Part model, mm, in its own coordinate system. A direction names the side the tool comes from. Round coordinates to 2 decimals unless told otherwise and drop trailing zeros. Loops run counter-clockwise (first coordinate to the right, second up) from the corner with the lowest first, then second, coordinate; pieces in that order, holes last. Notation, with made-up numbers: M -37,73 L -1,73 A6 ccw -1,79 Z; hole C 54,43 d10. An arc over 180 degrees is marked long. Put each result on its own line as item: value. Start each with the question number.
1) Slice it at A-A on y = 25.5. Give the cut face in (x, z) (3 decimals).
2) Slice it at C-C on z = 19.5. Give the cut face in (x, y), then the cut area to 3 significant figures.
3) Drop flat-ended pins along their axis: pin 1 Ø2 at (y, z) = (-5, 16.5) entering from +X; pin 2 Ø5 at (x, y) = (-6.5, 16) entering from +Z (3 decimals); pin 3 Ø1.1 at (y, z) = (25, 14.5) entering from -X (3 decimals). Give the stop position or say it passes through.
4) Which spindle directions (+Z, -Z, +X, -X, +Y, -Y) get a long thin tool onto all of the face, cutting with end or side? Do faces 4 (the flat face through (10.671, 6, 5)), 5 (the flat face through (-3.81, -5, 16)), 6 (the flat face through (-8.255, 25, 13)), 7 (the cylindrical face through (9.592, 25.453, 8.452)), 8 (the cylindrical face through (-7.205, -4.454, 13.832)). Say none if no direction does.
5) Pull direction Y, two halves, no side cores. Call faces 1 (the cylindrical face through (0.14, 25.41, 12.07)), 2 (the cylindrical face through (2.736, 23.264, 21.839)), 3 (the flat face through (0, 29.21, 6)): +Y half, -Y half, draft (parallel to the pull), parting line (faces both ways), or undercut.
6) Probe line 1 along Y through (x, z) = (8.5, 4.25); line 2 along Y through (x, z) = (6.35, 2.25); line 3 along X through (y, z) = (26, 15.25) (3 decimals). List the from-to ranges inside material, lowest first.
7) Slice it at D-D on y = 21. Give the cut face in (x, z) (3 decimals).
8) Slice it at B-B on y = 5. Give the cut face in (x, z) (3 decimals).
```python
from build123d import *

# Parameters (mm, degrees)
SKETCH1_W           = 25.4
SKETCH1_H           = 35.56
SKETCH1_R           = 2.38125
BOSS_EXTRUDE1_DEPTH = 3.175
SKETCH7_W           = 25.4
SKETCH7_H           = 2.54
SKETCH7_H_2         = 7.62
BOSS_EXTRUDE3_DEPTH = 20.32
SKETCH11_R          = 1.5875
CUT_EXTRUDE1_DEPTH  = 10
CHAMFER2_SIZE       = 1.27
SKETCH13_R          = 3.175
CUT_EXTRUDE2_DEPTH  = 12.7
SKETCH14_R          = 7.14375
CUT_EXTRUDE3_DEPTH  = 3.302
CUT_EXTRUDE4_START  = -3.302
SKETCH15_R          = 7.14375
CUT_EXTRUDE4_DEPTH  = 3.302
CUT_EXTRUDE5_DEPTH  = 12.7
SKETCH17_W          = 2.029010409
SKETCH17_H          = 25.4
BOSS_EXTRUDE4_DEPTH = 12.7
CUT_EXTRUDE6_DEPTH  = 46.281333074


with BuildPart() as part:
    # Sketch1 → Boss-Extrude1 (new body)
    with BuildSketch(Plane.XY):
        with Locations((0, 11.43)):
            Rectangle(SKETCH1_W, SKETCH1_H)
        with Locations((-6.35, 3.175)):
            Circle(SKETCH1_R, mode=Mode.SUBTRACT)
        with Locations(Location((6.35, 3.175, 0), (0, 0, 180))):
            Circle(SKETCH1_R, mode=Mode.SUBTRACT)
    extrude(amount=BOSS_EXTRUDE1_DEPTH)

    # Sketch7 → Boss-Extrude3 (add)
    with BuildSketch(Plane.XY.offset(3.175)):
        with Locations((0, -5.08)):
            Rectangle(SKETCH7_W, SKETCH7_H)
        with Locations((0, 25.4)):
            Rectangle(SKETCH7_W, SKETCH7_H_2)
    extrude(amount=BOSS_EXTRUDE3_DEPTH)

    # Sketch11 → Cut-Extrude1 (cut)
    with BuildSketch(Plane.XZ.offset(6.35)):
        with Locations((-7.9375, 15.24)):
            Circle(SKETCH11_R)
        with Locations((7.9375, 15.24)):
            Circle(SKETCH11_R)
        with Locations((0, 5.715)):
            Circle(SKETCH11_R)
        with BuildLine():
            Line((-3.814625586, 12.241539102), (-3.814692285, 12.218981082))
            ThreePointArc((-3.814692285, 12.218981082), (0, 8.404288797), (3.814692285, 12.218981082))
            Line((3.814692285, 12.218981082), (3.814625586, 12.241539102))
            Line((3.814625586, 12.241539102), (3.81, 13.805952441))
            Line((3.81, 13.805952441), (3.81, 17.615952441))
            ThreePointArc((3.81, 17.615952441), (9.167172212, 19.841012117), (12.7, 15.24))
            Line((12.7, 15.24), (12.7, 23.495))
            Line((12.7, 23.495), (-12.7, 23.495))
            Line((-12.7, 23.495), (-12.7, 15.24))
            ThreePointArc((-12.7, 15.24), (-9.167172212, 19.841012117), (-3.81, 17.615952441))
            Line((-3.81, 17.615952441), (-3.81, 13.805952441))
            Line((-3.81, 13.805952441), (-3.814625586, 12.241539102))
        make_face()
    extrude(amount=-CUT_EXTRUDE1_DEPTH, mode=Mode.SUBTRACT)

    # Chamfer2
    # the kernel refuses this chamfer: 1.27 mm, written as the material it takes off along each edge
    with BuildSketch(Plane(origin=(-7.9375, -6.35, 15.24), x_dir=(1, 0, 0), z_dir=(0, 0, -1))) as chamfer2_piece_1:
        Polygon((1.5875 + CHAMFER2_SIZE, 0), (1.5875, -CHAMFER2_SIZE), (1.5875, 0), align=None)
    revolve(axis=Axis((-7.9375, -6.35, 15.24), (0, -1, 0)), mode=Mode.SUBTRACT)
    with BuildSketch(Plane(origin=(7.9375, -6.35, 15.24), x_dir=(1, 0, 0), z_dir=(0, 0, -1))) as chamfer2_piece_2:
        Polygon((1.5875 + CHAMFER2_SIZE, 0), (1.5875, -CHAMFER2_SIZE), (1.5875, 0), align=None)
    revolve(axis=Axis((7.9375, -6.35, 15.24), (0, -1, 0)), mode=Mode.SUBTRACT)
    with BuildSketch(Plane(origin=(0, -6.35, 5.715), x_dir=(1, 0, 0), z_dir=(0, 0, -1))) as chamfer2_piece_3:
        Polygon((1.5875 + CHAMFER2_SIZE, 0), (1.5875, -CHAMFER2_SIZE), (1.5875, 0), align=None)
    revolve(axis=Axis((0, -6.35, 5.715), (0, -1, 0)), mode=Mode.SUBTRACT)

    # Sketch13 → Cut-Extrude2 (cut)
    with BuildSketch(Plane(origin=(0, 29.21, 0), x_dir=(1, 0, 0), z_dir=(0, 1, 0))):
        with Locations(Location((0, -15.24, 0), (0, 0, 270))):
            Circle(SKETCH13_R)
    extrude(amount=-CUT_EXTRUDE2_DEPTH, mode=Mode.SUBTRACT)

    # Sketch14 → Cut-Extrude3 (cut)
    with BuildSketch(Plane(origin=(0, 29.21, 0), x_dir=(1, 0, 0), z_dir=(0, 1, 0))):
        with Locations(Location((0, -15.24, 0), (0, 0, 270))):
            Circle(SKETCH14_R)
    extrude(amount=-CUT_EXTRUDE3_DEPTH, mode=Mode.SUBTRACT)

    # Sketch15 → Cut-Extrude4 (cut)
    with BuildSketch(Plane.XZ.offset(-21.59).offset(CUT_EXTRUDE4_START)):
        with Locations(Location((0, 15.24, 0), (0, 0, 90))):
            Circle(SKETCH15_R)
    extrude(amount=CUT_EXTRUDE4_DEPTH, mode=Mode.SUBTRACT)

    # Sketch16 → Cut-Extrude5 (cut)
    with BuildSketch(Plane(origin=(0, 29.21, 0), x_dir=(1, 0, 0), z_dir=(0, 1, 0))):
        with BuildLine():
            ThreePointArc((8.255, -15.24), (5.837166479, -21.077166479), (0, -23.495))
            Line((0, -23.495), (12.7, -23.495))
            Line((12.7, -23.495), (12.7, -7.184415797))
            ThreePointArc((12.7, -7.184415797), (9.556910358, -8.486326154), (8.255, -11.629415797))
            Line((8.255, -11.629415797), (8.255, -15.24))
        make_face()
        with BuildLine():
            ThreePointArc((0, -23.495), (-5.837166479, -21.077166479), (-8.255, -15.24))
            Line((-8.255, -15.24), (-8.255, -11.629415797))
            ThreePointArc((-8.255, -11.629415797), (-9.556910358, -8.486326154), (-12.7, -7.184415797))
            Line((-12.7, -7.184415797), (-12.7, -23.495))
            Line((-12.7, -23.495), (0, -23.495))
        make_face()
    extrude(amount=-CUT_EXTRUDE5_DEPTH, mode=Mode.SUBTRACT)

    # Sketch17 → Boss-Extrude4 (add)
    with BuildSketch(Plane.XY.offset(3.175)):
        with Locations((-11.685494796, 8.89)):
            Rectangle(SKETCH17_W, SKETCH17_H)
        with Locations((11.685494796, 8.89)):
            Rectangle(SKETCH17_W, SKETCH17_H)
    extrude(amount=BOSS_EXTRUDE4_DEPTH)

    # Sketch18 → Cut-Extrude6 (cut, through all)
    with BuildSketch(Plane(origin=(12.7, 0, 0), x_dir=(0, 0, -1), z_dir=(1, 0, 0))):
        with BuildLine():
            ThreePointArc((-7.184415797, 21.59), (-5.951695656, 7.221633885), (-15.24, -3.81))
            Line((-15.24, -3.81), (-15.875, -3.81))
            Line((-15.875, -3.81), (-15.875, 21.59))
            Line((-15.875, 21.59), (-7.184415797, 21.59))
        make_face()
    extrude(amount=-CUT_EXTRUDE6_DEPTH, mode=Mode.SUBTRACT)


solid = part.part
```
Recorded:
1. outline: M -12.7,0 L 12.7,0 L 12.7,7.184 A4.445 cw 8.255,11.629 L 8.255,15.24 A8.255 ccw -8.255,15.24 L -8.255,11.629 A4.445 cw -12.7,7.184 Z; hole C 0,15.24 d6.35
2. outline: M -10.07,-6.35 L -5.81,-6.35 L -5.81,-3.81 L -10.07,-3.81 Z; M -7.07,21.59 L -5.73,21.59 L -5.73,24.89 L 5.73,24.89 L 5.73,21.59 L 7.07,21.59 L 7.07,29.21 L 5.73,29.21 L 5.73,25.91 L -5.73,25.91 L -5.73,29.21 L -7.07,29.21 Z; M 5.81,-6.35 L 10.07,-6.35 L 10.07,-3.81 L 5.81,-3.81 Z
2. area: 53.7 mm2
3. pin 1: stops at x = 12.69
3. pin 2: stops at z = 3.175
3. pin 3: stops at x = -8.255
4. face 4: +Z
4. face 5: +Z, -Y
4. face 6: +Z, -X, +Y
4. face 7: +Z, +X, +Y
4. face 8: -Y
5. face 1: draft
5. face 2: undercut
5. face 3: +Y half
6. line 1: y = -6.35 to -3.81, 21.59 to 29.21
6. line 2: y = -6.35 to 0.79, 5.56 to 29.21
6. line 3: x = -8.255 to -7.144, 7.144 to 8.255
7. outline: M -12.7,0 L 12.7,0 L 12.7,6.892 L 10.671,6.892 L 10.671,3.175 L -10.671,3.175 L -10.671,6.892 L -12.7,6.892 Z
8. outline: M -12.7,0 L -7.88,0 L -7.88,3.175 L -10.671,3.175 L -10.671,6.814 L -12.7,6.814 Z; M -4.82,0 L 4.82,0 L 4.82,3.175 L -4.82,3.175 Z; M 7.88,0 L 12.7,0 L 12.7,6.814 L 10.671,6.814 L 10.671,3.175 L 7.88,3.175 Z
